from build123d import *

# Parameters (mm, degrees)
SKETCH009_R        = 16.5
SKETCH009_R_2      = 2
PAD006_DEPTH       = 3
SKETCH010_R        = 1.5
PAD007_DEPTH       = 25
POLARPATTERN_COUNT = 9
PAD008_DEPTH       = 25
SKETCH012_R        = 21.5
SKETCH012_R_2      = 18.7
SKETCH012_R_3      = 2.1
PAD009_DEPTH       = 2
PAD010_DEPTH       = 8.5
SKETCH014_R        = 2.8
PAD011_DEPTH       = 2.6


with BuildPart() as part:
    # Sketch009 → Pad006 (new body)
    with BuildSketch(Plane.YZ):
        Circle(SKETCH009_R)
        with Locations((0, 12)):
            Circle(SKETCH009_R_2, mode=Mode.SUBTRACT)
        with Locations((-6, 10.392305)):
            Circle(SKETCH009_R_2, mode=Mode.SUBTRACT)
        with Locations((6, 10.392305)):
            Circle(SKETCH009_R_2, mode=Mode.SUBTRACT)
        with Locations((12, 0)):
            Circle(SKETCH009_R_2, mode=Mode.SUBTRACT)
        with Locations((10.392305, -6)):
            Circle(SKETCH009_R_2, mode=Mode.SUBTRACT)
        with Locations((6, -10.392305)):
            Circle(SKETCH009_R_2, mode=Mode.SUBTRACT)
        with Locations((-6, -10.392305)):
            Circle(SKETCH009_R_2, mode=Mode.SUBTRACT)
        with Locations((-10.392305, -6)):
            Circle(SKETCH009_R_2, mode=Mode.SUBTRACT)
        with Locations((-12, 0)):
            Circle(SKETCH009_R_2, mode=Mode.SUBTRACT)
    extrude(amount=PAD006_DEPTH)

    # Sketch010 → Pad007 (join)
    with BuildSketch(Plane.YZ):
        with BuildLine():
            ThreePointArc((5.510568, -35.069697), (0, 35.5), (-5.510568, -35.069697))
            ThreePointArc((-2.988125, -37.766667), (-3.785221, -35.984091), (-5.510568, -35.069697))
            ThreePointArc((-2.988125, -37.766667), (0, -40.5), (2.988125, -37.766667))
            ThreePointArc((5.510568, -35.069697), (3.785221, -35.984091), (2.988125, -37.766667))
        make_face()
        with Locations((0, -37.5)):
            Circle(SKETCH010_R, mode=Mode.SUBTRACT)
    pad007 = extrude(amount=-PAD007_DEPTH)

    # PolarPattern: Pad007 ×9 about axis
    polarpattern_axis = Axis((0, 0, 0), (1, 0, 0))
    for i in range(1, POLARPATTERN_COUNT):
        add(pad007.rotate(polarpattern_axis, i * 360 / POLARPATTERN_COUNT))

    # Sketch011 → Pad008 (join)
    with BuildSketch(Plane.YZ):
        with BuildLine():
            ThreePointArc((-6.626667, 34.876027), (-5.459437, 35.565466), (-5, 36.840874))
            Line((-5, 37.840874), (-5, 36.840874))
            ThreePointArc((-3, 39.840874), (-4.414214, 39.255088), (-5, 37.840874))
            Line((-3, 39.840874), (3, 39.840874))
            ThreePointArc((5, 37.840874), (4.414214, 39.255088), (3, 39.840874))
            Line((5, 37.840874), (5, 36.840874))
            ThreePointArc((5, 36.840874), (5.459437, 35.565466), (6.626667, 34.876027))
            ThreePointArc((6.626667, 34.876027), (0, 35.5), (-6.626667, 34.876027))
        make_face()
    extrude(amount=-PAD008_DEPTH)

    # Sketch012 → Pad009 (join)
    with BuildSketch(Plane.YZ):
        Circle(SKETCH012_R)
        Circle(SKETCH012_R_2, mode=Mode.SUBTRACT)
        with Locations((0, 29)):
            Circle(SKETCH012_R_3)
    extrude(amount=PAD009_DEPTH)

    # Sketch013 → Pad010 (join)
    with BuildSketch(Plane.YZ.offset(-25)):
        with BuildLine():
            ThreePointArc((-7, 30.712375), (0, -31.5), (7, 30.712375))
            Line((7, 36.5), (7, 30.712375))
            Line((-7, 36.5), (7, 36.5))
            Line((-7, 30.712375), (-7, 36.5))
        make_face()
    extrude(amount=-PAD010_DEPTH)

    # Sketch014 → Pad011 (join)
    with BuildSketch(Plane.YZ.offset(-25)):
        Circle(SKETCH014_R)
        with Locations((0, -37.5)):
            Circle(SKETCH014_R)
        with Locations((-32.475953, 18.75)):
            Circle(SKETCH014_R)
    extrude(amount=-PAD011_DEPTH)


with BuildPart() as part_1:
    # Body004 placement: moved
    add(part.part.moved(Location((107.2, 0, 107))))


solid = part_1.part
Work out the finished part from the listing and answer in its coordinate system (mm). A direction names the side the tool comes from. Give positions to 0.01 mm unless a question says otherwise; leave off trailing zeros. Write each loop counter-clockwise with the first axis right and the second up, starting at its lowest first coordinate (ties: lowest second). Pieces come first, ordered by that corner, then holes.
Q1. A tool of negligible diameter and unlimited length cuts with its end or side. For faces 1 (the face through (94.875, 12.051, 73.608)), 2 (the face through (94.875, 0.806, 70.765)), 3 (the face through (94.88, 5.45, 142.58)), 4 (the face through (94.875, -38.121, 99.575)), 5 (the face through (82.2, 23.5, 85.6)), from which of +Z, -Z, +X, -X, +Y, -Y can it reach the whole face along a straight path? Write none if from no direction.
Answer:
face 1: -Z, +X, -X
face 2: +X
face 3: +Z, +X
face 4: +X, -X
face 5: -X
Q2. For a pull along Y with two mould halves and no side action, classify faces 6 (the face through (94.875, 22.892, 134.133)), 7 (the face through (109.2, 0, 136)), 8 (the face through (80.92, -34.54, 127.64)) as released by +Y, released by -Y, zero draft, split by the parting line, or undercut.
Answer:
face 6: released by +Y
face 7: zero draft
face 8: undercut
Q3. Straight lines are drawn through the part: L1, parallel to Z at x = 108, y = 0; L2, parallel to Y at x = 101, z = 78.5; L3, parallel to Y at x = 88, z = 143. For each, find the intervals that lie inside material, in ascending order.
Answer:
L1: z = 85.5 to 88.3, 90.5 to 117, 121 to 123.5, 125.7 to 128.5, 133.9 to 138.1
L2: y = -27.1 to -25.59, -22.62 to 22.62, 25.59 to 27.1
L3: y = -15.73 to -14.12, -11.53 to -9.8, -5.19 to 5.19, 9.8 to 11.53, 14.12 to 15.73
Q4. The part is cut by section B-B on y = -20. Give the vertices of the cut face in (x, z), and give its area (3 significant figures).
Answer:
outline: (73.7, 82.66) - (82.2, 82.66) - (82.2, 77.02) - (107.2, 77.02) - (107.2, 99.11) - (109.2, 99.11) - (109.2, 114.89) - (107.2, 114.89) - (107.2, 136.33) - (82.2, 136.33) - (82.2, 131.34) - (73.7, 131.34) - close
area: 1,930 mm2
Q5. The part is cut by section A-A on z = 139.5. Give the vertices of the cut face in (x, y), and give its area (3 significant figures).
Answer:
outline: (73.7, -7) - (82.2, -7) - (82.2, -15.87) - (107.2, -15.87) - (107.2, 15.87) - (82.2, 15.87) - (82.2, 7) - (73.7, 7) - close
area: 913 mm2
Q6. The part is cut by section C-C on z = 101. State how many separate pieces and enclosed holes the cut face has, and give its area (3 significant figures).
Answer:
separate pieces: 3
enclosed holes: 0
area: 2,460 mm2
Q7. Given pin 1 (1.8 mm diameter, centred on y = -36.93, z = 100.49, fed in from -X); pin 2 (5 mm diameter, centred on y = 29.5, z = 99.5, fed in from +X); pin 3 (12 mm diameter, centred on x = 90, z = 81, fed in from +Y); pin 4 (1.7 mm diameter, centred on y = 1, z = 70.5, fed in from -X), each flat-ended and moving along its own axis, determine where each tip first touches the part or whether it passes through.
Answer:
pin 1: passes through
pin 2: stops at x = 107.2
pin 3: stops at y = 29.33
pin 4: stops at x = 79.6
